Work out the finished part from the listing and answer in its coordinate system (mm). A direction names the side the tool comes from. Coordinates: 2 decimals unless noted, no trailing zeros. Write each loop counter-clockwise with the first axis right and the second up, starting at its lowest first coordinate (ties: lowest second). Pieces come first, ordered by that corner, then holes. Notation, with made-up numbers: (-11, -15) - (21, -15) arc R22 cw to (21, 4) - close; hole circle Ø5 at (58.5, 73). An arc over 180 degrees is marked (long way). Use one line per item in the form item = value. Start each with the question number.
Item 1: A cutting plane is placed at B-B (x = -14.5). Write down the section's boundary in (y, z).
Item 2: Given pin 1 (11 mm diameter, centred on y = 2, z = 13.5, fed in from +X); pin 2 (1.5 mm diameter, centred on y = -24, z = 4.5, fed in from -X); pin 3 (8 mm diameter, centred on y = 4.5, z = 8.5, fed in from -X), each flat-ended and moving along its own axis, determine where each tip first touches the part or whether it passes through.
Item 3: A cutting plane is placed at A-A (z = 3.5). Write down the section's boundary in (x, y), then the cut area to 3 significant figures.
Item 4: Determine the mould class of faces 1 (the flat face through (-34.592, 0, 13)), 2 (the flat face through (-27, -5, 25)), 3 (the flat face through (-27, -5, 0)), 4 (the flat face through (-26.592, 0, 1)) for opening direction Z: released by +Z, released by -Z, zero draft, split by the parting line, or undercut.
Item 5: Consider probe 1 along Z at (x, y) = (-30.25, 0); probe 2 along Y at (x, z) = (-20, 5.75); probe 3 along Y at (x, z) = (-10, 5.5). Determine where each line is inside the solid, lowest interval first.
Item 6: A cutting plane is placed at C-C (x = -29.5). Write down the section's boundary in (y, z).
Item 7: For faces 5 (the cylindrical face through (-30.54, 10.39, 8.19)), 6 (the flat face through (0, -34, 12)), determine the directions among +Z, -Z, +X, -X, +Y, -Y from which every point of the face is accessible in a straight line to the end or side of a thin tool.
Item 8: A cutting plane is placed at D-D (z = 12.5). Write down the section's boundary in (x, y).
from build123d import *

# Parameters (mm, degrees)
F1_DEPTH = 25
F2_R     = 11.25
F3_DEPTH = 8


with BuildPart() as f1:
    # F0 (on Top) → F1 (new body)
    with BuildSketch(Plane.XY):
        with BuildLine():
            ThreePointArc((0, -30), (-16.201852, -25.248762), (-27.27178, -12.5))
            Line((-27.27178, -12.5), (-26.592, -12.5))
            Line((-26.592, -12.5), (-26.592, 0))
            Line((-26.592, 0), (-26.592, 12.5))
            Line((-26.592, 12.5), (-27.27178, 12.5))
            ThreePointArc((-27.27178, 12.5), (-16.201852, 25.248762), (0, 30))
            Line((0, 30), (0, 37.5))
            ThreePointArc((0, 37.5), (-26.516504, 26.516504), (-37.5, 0))
            ThreePointArc((-37.5, 0), (-26.516504, -26.516504), (0, -37.5))
            Line((0, -37.5), (0, -30))
        make_face()
    extrude(amount=F1_DEPTH)

    # F2 (on face) → F3 (cut)
    with BuildSketch(Plane.YZ.offset(-26.592)):
        with Locations((0, 12.5)):
            Circle(F2_R)
    extrude(amount=-F3_DEPTH, mode=Mode.SUBTRACT)


solid = f1.part
Answer:
q1.outline = (-34.58, 0) - (-26.26, 0) - (-26.26, 25) - (-34.58, 25) - close; (26.26, 0) - (34.58, 0) - (34.58, 25) - (26.26, 25) - close
q2.pin_1 = -34.59
q2.pin_2 = -29.42
q2.pin_3 = -37.5
q3.outline = (-37.5, 0) arc R37.5 ccw to (0, -37.5) - (0, -30) arc R30 cw to (-27.27, -12.5) - (-26.59, -12.5) - (-26.59, -6.75) - (-34.59, -6.75) - (-34.59, 6.75) - (-26.59, 6.75) - (-26.59, 12.5) - (-27.27, 12.5) arc R30 cw to (0, 30) - (0, 37.5) arc R37.5 ccw to start
q3.area = 750 mm²
q4.face_1 = undercut
q4.face_2 = released by +Z
q4.face_3 = released by -Z
q4.face_4 = zero draft
q5.probe_1 = 0 to 1.25, 23.75 to 25
q5.probe_2 = -31.72 to -22.36, 22.36 to 31.72
q5.probe_3 = -36.14 to -28.28, 28.28 to 36.14
q6.outline = (-23.15, 0) - (23.15, 0) - (23.15, 25) - (-23.15, 25) - close; hole circle Ø22.5 at (0, 12.5)
q7.face_5 = +X
q7.face_6 = +Z, -Z, +X, +Y, -Y
q8.outline = (-37.5, 0) arc R37.5 ccw to (0, -37.5) - (0, -30) arc R30 cw to (-27.27, -12.5) - (-26.59, -12.5) - (-26.59, -11.25) - (-34.59, -11.25) - (-34.59, 11.25) - (-26.59, 11.25) - (-26.59, 12.5) - (-27.27, 12.5) arc R30 cw to (0, 30) - (0, 37.5) arc R37.5 ccw to start
